Input: part model. Units: mm. Frame: model coordinates. Face numbers are marked on the shaded views. A direction names the side the tool comes from. Coordinates: 2 decimals unless noted, no trailing zeros. Loops run counter-clockwise (first coordinate to the right, second up) from the corner with the lowest first, then second, coordinate; pieces in that order, holes last. Notation, with made-up numbers: (-18, 10.25) - (18, 10.25) arc R19 ccw to (18, 19.25) - close; hole circle Ø10 at (88.25, 67.25). An arc over 180 degrees is marked (long way). Use one line per item in the form item = value.
from build123d import *

# Parameters (mm, degrees)
F0_R     = 17.2417566051
F0_R_2   = 15.9851491333
F1_DEPTH = 25.4
F2_R     = 9.6526962005
F3_DEPTH = 35.814
F5_DEPTH = 635


with BuildPart() as f1:
    # F0 (on Top) → F1 (new body)
    with BuildSketch(Plane.XY):
        with BuildLine():
            ThreePointArc((-33.7519310415, -64.4190087914), (0, -98.1709398329), (33.7519310415, -64.4190087914))
            Line((33.7519310415, -64.4190087914), (33.7519310415, 64.4190087914))
            ThreePointArc((33.7519310415, 64.4190087914), (0, 98.1709398329), (-33.7519310415, 64.4190087914))
            Line((-33.7519310415, 64.4190087914), (-33.7519310415, -64.4190087914))
        make_face()
        with Locations((0, -64.4190087914)):
            Circle(F0_R, mode=Mode.SUBTRACT)
        with Locations((0, 64.4190087914)):
            Circle(F0_R_2, mode=Mode.SUBTRACT)
    extrude(amount=F1_DEPTH)

    # F2 (on Front) → F3 (join, symmetric)
    with BuildSketch(Plane.XZ):
        with BuildLine():
            Line((-17.2510873526, 24.3432018906), (17.2510873526, 24.3432018906))
            Line((17.2510873526, 24.3432018906), (17.2510873526, 74.9463941902))
            ThreePointArc((17.2510873526, 74.9463941902), (0, 92.1974815428), (-17.2510873526, 74.9463941902))
            Line((-17.2510873526, 74.9463941902), (-17.2510873526, 24.3432018906))
        make_face()
        with Locations((0, 74.9463941902)):
            Circle(F2_R, mode=Mode.SUBTRACT)
    extrude(amount=F3_DEPTH, both=True)

    # F4 (on Right) → F5 (cut, symmetric)
    with BuildSketch(Plane.YZ):
        with BuildLine():
            ThreePointArc((-14.9509394541, 50.0281564891), (0, 35.077217035), (14.9509394541, 50.0281564891))
            Line((14.9509394541, 50.0281564891), (-14.9509394541, 50.0281564891))
        make_face()
        with BuildLine():
            ThreePointArc((-14.9509394541, 50.0281564891), (0, 64.9790959433), (14.9509394541, 50.0281564891))
            Line((14.9509394541, 50.0281564891), (14.9509394541, 93.7309004366))
            Line((14.9509394541, 93.7309004366), (-14.9509394541, 93.7309004366))
            Line((-14.9509394541, 93.7309004366), (-14.9509394541, 50.0281564891))
        make_face()
        with BuildLine():
            Line((-14.9509394541, 50.0281564891), (14.9509394541, 50.0281564891))
            ThreePointArc((14.9509394541, 50.0281564891), (0, 64.9790959433), (-14.9509394541, 50.0281564891))
        make_face()
    extrude(amount=F5_DEPTH, both=True, mode=Mode.SUBTRACT)


solid = f1.part
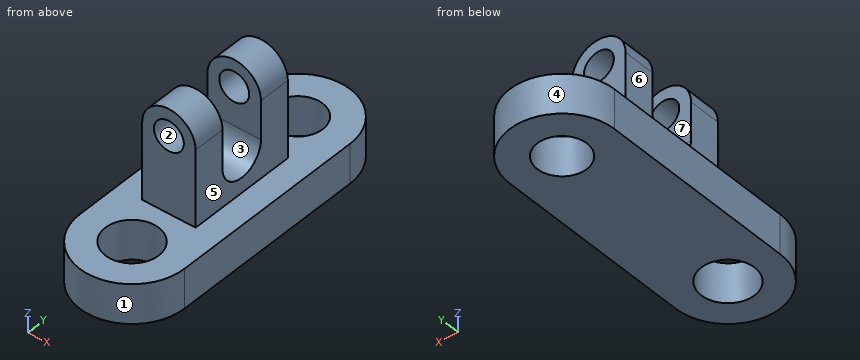
Q1. Cut plane B-B, the plane y = 24. Return loops of the section in (x, z), then the cut area to 3 significant figures.
Check values:
outline = (-33.75, 0) - (33.75, 0) - (33.75, 25.4) - (17.25, 25.4) - (17.25, 74.95) arc R17.25 ccw to (-17.25, 74.95) - (-17.25, 25.4) - (-33.75, 25.4) - close; hole circle Ø19.31 at (0, 74.95)
area = 3,600 mm²
Q2. Pull-direction query (Y, two-part tool) for the marked faces 1, 2, 3 and 4; classes: pulls with the +Y half, pulls with the -Y half, needs draft (parallel to the pull), parting line crosses it, or undercut.
Check values:
face_1 = pulls with the -Y half
face_2 = needs draft
face_3 = undercut
face_4 = pulls with the +Y half
Q3. Ray query, line 1 along Y through (x, z) = (0, 13.5); line 2 along Z through (x, y) = (0, 28.75); line 3 along Y through (x, z) = (-15, 75). Return the intervals inside material, ascending. Write a range as [from, to].
Check values:
line_1 = [-98.17, -81.66], [-47.18, 48.43], [80.4, 98.17]
line_2 = [0, 65.29], [84.6, 92.2]
line_3 = [-35.81, -14.95], [14.95, 35.81]
Q4. First-contact query: P1, Ø1, axis at x = -7.5, z = 19, coming from the -Y side; P2, Ø2, axis at x = 6, z = 29.5, coming from the +Y side; P3, Ø6, axis at x = -21.5, z = 65, coming from the -Y side; P4, Ø1.5, axis at y = 35.5, z = 28, coming from the +X side. Flat tips, straight axial feed; report the tip coordinate or a pass-through.
Check values:
P1 = -97.44
P2 = 35.81
P3 = through
P4 = 17.25
Q5. Set-up query: the marked faces 5, 6 and 7. Return all of +Z, -Z, +X, -X, +Y, -Y with unobstructed straight access to the full face (end or side cutting, diameter ignored); none if empty.
Check values:
face_5 = +Z, +X, +Y, -Y
face_6 = +Z, -X, +Y, -Y
face_7 = +Z, +X, -X
Q6. Cut plane A-A, the plane x = 0. Return loops of the section in (y, z).
Check values:
outline = (-98.17, 0) - (-81.66, 0) - (-81.66, 25.4) - (-98.17, 25.4) - close; (-47.18, 0) - (48.43, 0) - (48.43, 25.4) - (35.81, 25.4) - (35.81, 65.29) - (14.95, 65.29) - (14.95, 50.03) arc R14.95 cw to (-14.95, 50.03) - (-14.95, 65.29) - (-35.81, 65.29) - (-35.81, 25.4) - (-47.18, 25.4) - close; (-35.81, 84.6) - (-14.95, 84.6) - (-14.95, 92.2) - (-35.81, 92.2) - close; (14.95, 84.6) - (35.81, 84.6) - (35.81, 92.2) - (14.95, 92.2) - close; (80.4, 0) - (98.17, 0) - (98.17, 25.4) - (80.4, 25.4) - close
Q7. Cut plane C-C, the plane z = 86.5. Return loops of the section in (x, y), then the cut area to 3 significant figures.
Check values:
outline = (-12.81, -35.81) - (12.81, -35.81) - (12.81, -14.95) - (-12.81, -14.95) - close; (-12.81, 14.95) - (12.81, 14.95) - (12.81, 35.81) - (-12.81, 35.81) - close
area = 1,070 mm²
Q8. Cut plane D-D, the plane x = 13.5. Return loops of the section in (y, z).
Check values:
outline = (-95.35, 0) - (-75.14, 0) - (-75.14, 25.4) - (-95.35, 25.4) - close; (-53.69, 0) - (55.86, 0) - (55.86, 25.4) - (35.81, 25.4) - (35.81, 85.69) - (14.95, 85.69) - (14.95, 50.03) arc R14.95 cw to (-14.95, 50.03) - (-14.95, 85.69) - (-35.81, 85.69) - (-35.81, 25.4) - (-53.69, 25.4) - close; (72.98, 0) - (95.35, 0) - (95.35, 25.4) - (72.98, 25.4) - close
